Build history of the part. All positions in model axes, mm. Round coordinates to 2 decimals unless told otherwise and drop trailing zeros. Write each loop counter-clockwise with the first axis right and the second up, starting at its lowest first coordinate (ties: lowest second). Pieces come first, ordered by that corner, then holes.
from build123d import *

# Parameters (mm, degrees)
SKETCH1_R               = 35.5406
BOSS_EXTRUDE1_DEPTH     = 140
CUT_EXTRUDE1_DEPTH      = 285.475426877
CUT_EXTRUDE1_DEPTH_BACK = 285.475426877
SKETCH3_R               = 4.131775048


with BuildPart() as part:
    # Sketch1 → Boss-Extrude1 (new, symmetric)
    with BuildSketch(Plane.XY):
        Circle(SKETCH1_R)
    extrude(amount=BOSS_EXTRUDE1_DEPTH, both=True)

    # Sketch3 → Cut-Extrude1 (cut, two sides: drawn at the far end of the back side and taken through both)
    with BuildSketch(Plane.XY.offset(140).offset(-CUT_EXTRUDE1_DEPTH_BACK)):
        with Locations((-15.363902822, 14.74340124)):
            Circle(SKETCH3_R)
        with Locations((15.363902822, 14.74340124)):
            Circle(SKETCH3_R)
        with BuildLine():
            ThreePointArc((-21.71870656, -8.592271503), (0, -23.356569616), (21.71870656, -8.592271503))
            ThreePointArc((21.71870656, -8.592271503), (0, -27.784875685), (-21.71870656, -8.592271503))
        make_face()
    extrude(amount=CUT_EXTRUDE1_DEPTH + CUT_EXTRUDE1_DEPTH_BACK, mode=Mode.SUBTRACT)


solid = part.part
1) Slice it at A-A (x = 0). Write the cut outline in (y, z), plus the area to 3 significant figures.
Results:
outline: (-35.54, -140) - (-27.78, -140) - (-27.78, 140) - (-35.54, 140) - close; (-23.36, -140) - (35.54, -140) - (35.54, 140) - (-23.36, 140) - close
area: 18,700 mm2
2) Mould opens along X. For faces 1 (the flat face through (0, 0, 140)), 2 (the cylindrical face through (0.44, -27.78, -1.96)), 3 (the cylindrical face through (-7.705, -34.695, 1.96)) say: released by +X, released by -X, zero draft, split by the parting line, or undercut.
Results:
face 1: zero draft
face 2: undercut
face 3: split by the parting line
3) Slice it at B-B (y = -20). Write the cut outline in (x, z).
Results:
outline: (-29.38, -140) - (-16.74, -140) - (-16.74, 140) - (-29.38, 140) - close; (-12.06, -140) - (12.06, -140) - (12.06, 140) - (-12.06, 140) - close; (16.74, -140) - (29.38, -140) - (29.38, 140) - (16.74, 140) - close
4) Pin check, flat tips, straight feed: pin 1 Ø6.5 at (x, y) = (15.36, 14.74) entering from -Z; pin 2 Ø4 at (x, z) = (11.5, 34.5) entering from +Y; pin 3 Ø2 at (x, z) = (-19, 24.5) entering from +Y; pin 4 Ø1 at (x, z) = (21.5, 25.5) entering from -Y. Stop position of each tip, or through.
Results:
pin 1: passes through
pin 2: stops at y = 34.25
pin 3: stops at y = 30.65
pin 4: stops at y = -28.67
5) Slice it at D-D (y = 27.5). Write the cut outline in (x, z).
Results:
outline: (-22.51, -140) - (22.51, -140) - (22.51, 140) - (-22.51, 140) - close
6) Wall check: L1, parallel to Y at x = 18, z = -91 (3 decimals); L2, parallel to Y at x = 1.5, z = 43.5; L3, parallel to Y at x = -17, z = 110.5. Give the ranges that are in metal, low to high.
Results:
L1: y = -30.645 to -18.348, -14.884 to 11.562, 17.925 to 30.645
L2: y = -35.51 to -27.73, -23.31 to 35.51
L3: y = -31.21 to -19.68, -16.02 to 10.95, 18.54 to 31.21
7) Slice it at C-C (z = 46). Write the cut outline in (x, y), plus the area to 3 significant figures.
Results:
outline: circle Ø71.08 at (0, 0); hole (-21.72, -8.59) arc R21.88 ccw to (21.72, -8.59) arc R23.36 cw to start; hole circle Ø8.26 at (-15.36, 14.74); hole circle Ø8.26 at (15.36, 14.74)
area: 3,690 mm2
